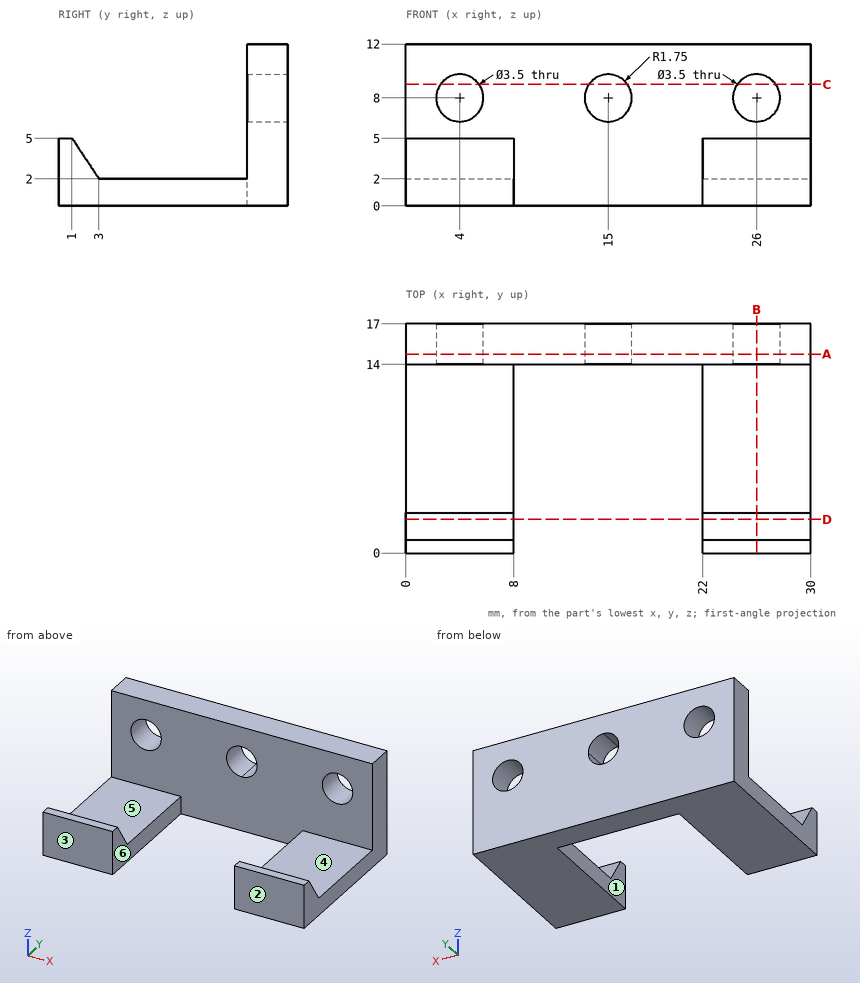
Can you work these out from the drawing? Everything is in mm from the part's minimum corner. A direction names the side the tool comes from. Give positions to 0.01 mm unless a question says otherwise; leave off trailing zeros. Write each loop counter-clockwise with the first axis right and the second up, starting at its lowest first coordinate (ties: lowest second). Pieces come first, ordered by that corner, then holes. Notation, with made-up numbers: M 82,85 L 130,85 A11 cw 130,93 Z; hole C 62.5,29.25 d8. An arc over 180 degrees is marked long. Answer in a Markdown table with one row per item. Add a question column.
Item 1: Imagine slicing it at A-A, the plane y = 14.75. Write out the boundary of the cut face in (x, z).
Item 2: On a 3-axis mill with a long thin cutter (end or side, diameter ignored), from which of +Z, -Z, +X, -X, +Y, -Y can I reach the whole of each face in a straight line? I mean the marked faces 1 and 2. Say none if no direction works.
Item 3: Imagine slicing it at B-B, the plane x = 26. Write out the boundary of the cut face in (y, z), plus the area to 3 significant figures.
Item 4: Please list where these lines run through material, in increasing order: L1, parallel to Y at x = 23.75, z = 3.5; L2, parallel to Z at x = 26, y = 14.95; L3, parallel to X at y = 8, z = 1.
Item 5: Imagine slicing it at D-D, the plane y = 2.5. Write out the boundary of the cut face in (x, z), plus the area to 3 significant figures.
Item 6: Imagine slicing it at C-C, the plane z = 9. Write out the boundary of the cut face in (x, y), plus the area to 3 significant figures.
Item 7: For pin 1 Ø4 at (x, y) = (2, 7) entering from +Z; pin 2 Ø0.8 at (x, y) = (3.5, 0.5) entering from +Z; pin 3 Ø3.5 at (x, z) = (17.5, 8) entering from -Y, each with a flat end and sliding along its axis, tell me the tip position at first contact or that it passes through.
Item 8: We'd pull the mould along Y, two halves only. Please class the marked faces 3, 4, 5 and 6: released by +Y, released by -Y, zero draft, split by the parting line, or undercut.
Evaluation:
| question | item | result |
|---|---|---|
| 1 | outline | M 0,0 L 30,0 L 30,12 L 0,12 Z; hole C 4,8 d3.5; hole C 15,8 d3.5; hole C 26,8 d3.5 |
| 2 | face 1 | +Z, -Z, -Y |
| 2 | face 2 | +Z, -Z, +X, -X, -Y |
| 3 | outline | M 0,0 L 17,0 L 17,6.25 L 14,6.25 L 14,2 L 3,2 L 1,5 L 0,5 Z; M 14,9.75 L 17,9.75 L 17,12 L 14,12 Z |
| 3 | area | 59.5 mm² |
| 4 | L1 | y = 0 to 2, 14 to 17 |
| 4 | L2 | z = 0 to 6.25, 9.75 to 12 |
| 4 | L3 | x = 0 to 8, 22 to 30 |
| 5 | outline | M 0,0 L 8,0 L 8,2.75 L 0,2.75 Z; M 22,0 L 30,0 L 30,2.75 L 22,2.75 Z |
| 5 | area | 44.0 mm² |
| 6 | outline | M 0,14 L 2.56,14 L 2.56,17 L 0,17 Z; M 5.44,14 L 13.56,14 L 13.56,17 L 5.44,17 Z; M 16.44,14 L 24.56,14 L 24.56,17 L 16.44,17 Z; M 27.44,14 L 30,14 L 30,17 L 27.44,17 Z |
| 6 | area | 64.1 mm² |
| 7 | pin 1 | stops at z = 2 |
| 7 | pin 2 | stops at z = 5 |
| 7 | pin 3 | stops at y = 14 |
| 8 | face 3 | released by -Y |
| 8 | face 4 | undercut |
| 8 | face 5 | undercut |
| 8 | face 6 | zero draft |
